The listing builds one solid part. Answer for the finished solid, in the listing's coordinates (mm). Face numbers are marked on the shaded views. A direction names the side the tool comes from. Give positions to 0.01 mm unless a question says otherwise; leave off trailing zeros. Order: outer loops, then holes, each group sorted by start corner. A loop starts at its lowest first (then second) coordinate and runs counter-clockwise, first axis right, second up.
```python
from build123d import *

# Parameters (mm, degrees)
SKETCH2_R           = 10
BOSS_EXTRUDE1_DEPTH = 30
SKETCH3_R           = 30
SKETCH3_R_2         = 15
BOSS_EXTRUDE2_DEPTH = 50
SKETCH3_3_R         = 15
BOSS_EXTRUDE3_DEPTH = 200
FILLET1_R           = 10
SCALE1_SCALE        = 0.3


with BuildPart() as part:
    # Sketch2 → Boss-Extrude1 (new body)
    with BuildSketch(Plane.XZ.offset(245.071627094)):
        with BuildLine():
            Line((57.282196187, 25), (90, 25))
            ThreePointArc((90, 25), (115, 0), (90, -25))
            Line((90, -25), (57.282196187, -25))
            ThreePointArc((57.282196187, -25), (44.194173824, -44.194173824), (25, -57.282196187))
            Line((25, -57.282196187), (25, -90))
            ThreePointArc((25, -90), (0, -115), (-25, -90))
            Line((-25, -90), (-25, -57.282196187))
            ThreePointArc((-25, -57.282196187), (-44.194173824, -44.194173824), (-57.282196187, -25))
            Line((-57.282196187, -25), (-90, -25))
            ThreePointArc((-90, -25), (-115, 0), (-90, 25))
            Line((-90, 25), (-57.282196187, 25))
            ThreePointArc((-57.282196187, 25), (-44.194173824, 44.194173824), (-25, 57.282196187))
            Line((-25, 57.282196187), (-25, 90))
            ThreePointArc((-25, 90), (0, 115.02832634), (25, 90))
            Line((25, 90), (25, 57.282196187))
            ThreePointArc((25, 57.282196187), (44.194173824, 44.194173824), (57.282196187, 25))
        make_face()
        with Locations((0, 90.028310311)):
            Circle(SKETCH2_R, mode=Mode.SUBTRACT)
        with Locations((90.028310311, 0.028310311)):
            Circle(SKETCH2_R, mode=Mode.SUBTRACT)
        with Locations((0.028310311, -90)):
            Circle(SKETCH2_R, mode=Mode.SUBTRACT)
        with Locations((-90, 0)):
            Circle(SKETCH2_R, mode=Mode.SUBTRACT)
    extrude(amount=BOSS_EXTRUDE1_DEPTH)

    # Sketch3 → Boss-Extrude2 (add)
    with BuildSketch(Plane.XZ.offset(275.071627094)):
        Circle(SKETCH3_R)
        Circle(SKETCH3_R_2, mode=Mode.SUBTRACT)
        Circle(SKETCH3_R_2)
    extrude(amount=BOSS_EXTRUDE2_DEPTH)

    # Sketch3_3 → Boss-Extrude3 (add)
    with BuildSketch(Plane.XZ.offset(275.071627094)):
        Circle(SKETCH3_3_R)
    extrude(amount=BOSS_EXTRUDE3_DEPTH)

    # Fillet1
    fillet1_edges = [part.edges().sort_by_distance(p)[0] for p in [
        (-15, -325.071627094, 0),
    ]]
    fillet(fillet1_edges, radius=FILLET1_R)


with BuildPart() as part_1:
    # Scale1: scaled about (-0.000611067, -283.723455746, 0.004725438)
    add(part.part.scale(SCALE1_SCALE).moved(Location((-0.000427747, -198.606419022, 0.003307807))))


solid = part_1.part
```
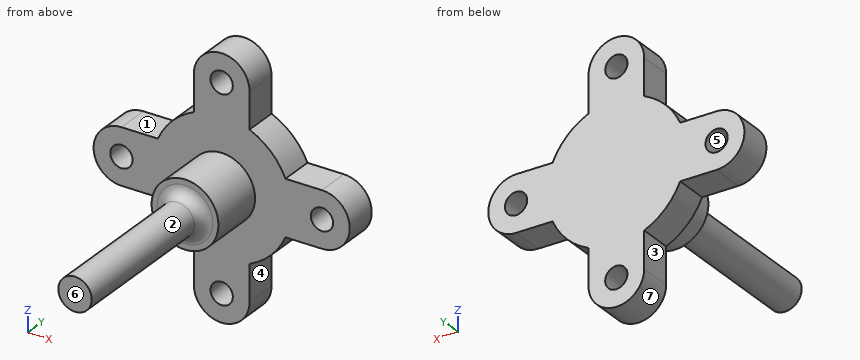
1) Given P1, Ø12, axis at y = -321.5, z = -15.5, coming from the -X side; P2, Ø4.5, axis at y = -276, z = -22, coming from the -X side; P3, Ø2.5, axis at y = -275, z = 20, coming from the +X side; P4, Ø12, axis at y = -314, z = -1.5, coming from the +X side, each flat-ended and moving along its own axis, determine where each tip first touches the part or whether it passes through.
Geometry says:
P1: passes through
P2: stops at x = -7.5
P3: stops at x = 7.5
P4: stops at x = 4.5
2) Find section D-D (y = -305). Write down the section's boundary in (x, z).
Geometry says:
outline: circle Ø9 at (0, 0)
3) A tool of negligible diameter and unlimited length cuts with its end or side. For the marked faces 1, 2, 3 and 4, from which of +Z, -Z, +X, -X, +Y, -Y can it reach the whole face along a straight path? Write none if from no direction.
Geometry says:
face 1: +Z, -X, +Y, -Y
face 2: -Y
face 3: -Z, -X, +Y, -Y
face 4: -Z, +X, +Y, -Y
4) Find section C-C (x = 21.5). Write down the section's boundary in (y, z).
Geometry says:
outline: (-281.13, -7.5) - (-272.13, -7.5) - (-272.13, 7.5) - (-281.13, 7.5) - close
5) Find section A-A (z = -25.5). Write down the section's boundary in (x, y).
Geometry says:
outline: (-7.5, -281.13) - (-2.59, -281.13) - (-2.59, -272.13) - (-7.5, -272.13) - close; (2.61, -281.13) - (7.5, -281.13) - (7.5, -272.13) - (2.61, -272.13) - close
6) Straight lines are drawn through the part: probe 1 along Y at (x, z) = (-3, 9); probe 2 along Y at (x, z) = (-3, 8); probe 3 along X at (y, z) = (-298.5, 2). For each, find the intervals that lie inside material, in ascending order.
Geometry says:
probe 1: y = -281.13 to -272.13
probe 2: y = -296.13 to -272.13
probe 3: x = -4.11 to 4.11
7) Find section B-B (y = -279.5). Write down the section's boundary in (x, z).
Geometry says:
outline: (-27, -7.5) - (-17.19, -7.5) arc R18.75 ccw to (-7.5, -17.18) - (-7.5, -27) arc R7.5 ccw to (7.5, -27) - (7.5, -17.18) arc R18.75 ccw to (17.18, -7.5) - (27, -7.5) arc R7.5 ccw to (27, 7.5) - (17.18, 7.5) arc R18.75 ccw to (7.5, 17.19) - (7.5, 27) arc R7.5 ccw to (-7.5, 27) - (-7.5, 17.19) arc R18.75 ccw to (-17.19, 7.5) - (-27, 7.5) arc R7.5 ccw to start; hole circle Ø6 at (-27, 0); hole circle Ø6 at (0, 27.01); hole circle Ø6 at (0.01, -27); hole circle Ø6 at (27.01, 0.01)
8) For a pull along X with two mould halves and no side action, classify the marked faces 5, 6 and 7 as +X half, -X half, draft (parallel to the pull), parting line (faces both ways), or undercut.
Geometry says:
face 5: undercut
face 6: draft
face 7: parting line
